Build history of the part. All positions in model axes, mm. Face numbers are marked on the shaded views. A direction names the side the tool comes from. Round coordinates to 2 decimals unless told otherwise and drop trailing zeros. Loops run counter-clockwise (first coordinate to the right, second up) from the corner with the lowest first, then second, coordinate; pieces in that order, holes last. Notation, with made-up numbers: (68, 27.25) - (95, 27.25) arc R23 cw to (95, 49.25) - close; hole circle Ø6 at (-33.75, -31.5). An arc over 180 degrees is marked (long way). Use a Markdown table: item, result.
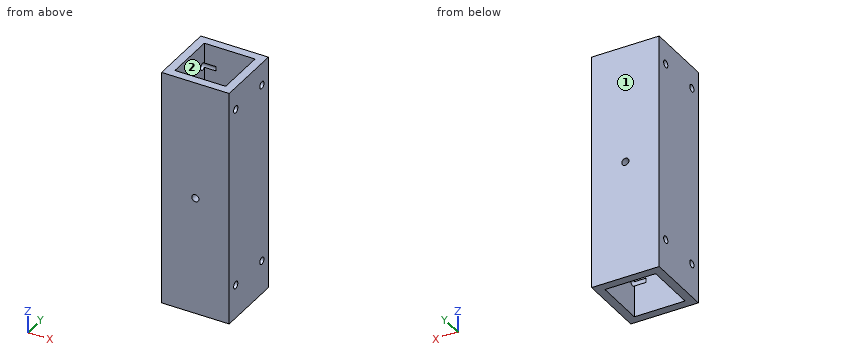
from build123d import *

# Parameters (mm, degrees)
SKETCH1_W                       = 38.1
SKETCH1_H                       = 133.35
BOSS_EXTRUDE1_DEPTH             = 19.05
SKETCH2_W                       = 28.575
SKETCH2_H                       = 28.575
CUT_EXTRUDE1_DEPTH              = 134.35
F_10_32_TAPPED_HOLE1_AT_2_COUNT = 2
F_10_32_TAPPED_HOLE1_AT_2_PITCH = 25.4
F_10_32_TAPPED_HOLE1_AT_3_COUNT = 2
F_10_32_TAPPED_HOLE1_AT_3_PITCH = 104.726882891
F_10_32_TAPPED_HOLE1_AT_4_COUNT = 2
F_10_32_TAPPED_HOLE1_AT_4_PITCH = 101.6
F_10_32_TAPPED_HOLE2_D          = 4.0386


with BuildPart() as part:
    # Sketch1 → Boss-Extrude1 (new body, symmetric)
    with BuildSketch(Plane(origin=(0, 0, 0), x_dir=(1, 0, 0), z_dir=(0, 1, 0))):
        Rectangle(SKETCH1_W, SKETCH1_H)
    extrude(amount=BOSS_EXTRUDE1_DEPTH, both=True)

    # Sketch2 → Cut-Extrude1 (cut, through all)
    with BuildSketch(Plane.XY.offset(66.675)):
        Rectangle(SKETCH2_W, SKETCH2_H)
    extrude(amount=-CUT_EXTRUDE1_DEPTH, mode=Mode.SUBTRACT)

    # Sketch3 → #10-32 Tapped Hole1 (revolve, cut)
    with BuildSketch(Plane(origin=(19.05, -12.7, 53.975), x_dir=(0, 0, -1), z_dir=(0, 1, 0))):
        Polygon((0, 0), (0, 12.389317848), (2.0193, 11.176), (2.0193, 0), align=None)
    f_10_32_tapped_hole1 = revolve(axis=Axis((25.4, -12.7, 53.975), (-1, 0, 0)), mode=Mode.SUBTRACT)

    # #10-32 Tapped Hole1 at 2: #10-32 Tapped Hole1 ×2
    with Locations(*[(0, i * F_10_32_TAPPED_HOLE1_AT_2_PITCH, 0) for i in range(1, F_10_32_TAPPED_HOLE1_AT_2_COUNT)]):
        add(f_10_32_tapped_hole1, mode=Mode.SUBTRACT)

    # #10-32 Tapped Hole1 at 3: #10-32 Tapped Hole1 ×2
    with Locations(*[Vector(0, 0.242535625, -0.9701425) * (i * F_10_32_TAPPED_HOLE1_AT_3_PITCH) for i in range(1, F_10_32_TAPPED_HOLE1_AT_3_COUNT)]):
        add(f_10_32_tapped_hole1, mode=Mode.SUBTRACT)

    # #10-32 Tapped Hole1 at 4: #10-32 Tapped Hole1 ×2
    with Locations(*[(0, 0, -i * F_10_32_TAPPED_HOLE1_AT_4_PITCH) for i in range(1, F_10_32_TAPPED_HOLE1_AT_4_COUNT)]):
        add(f_10_32_tapped_hole1, mode=Mode.SUBTRACT)

    # #10-32 Tapped Hole2 (through all)
    with Locations(Plane(origin=(0, 19.05, 0), x_dir=(1, 0, 0), z_dir=(0, 1, 0))):
        with Locations((0, 0)):
            Hole(F_10_32_TAPPED_HOLE2_D / 2)

    # Mirror1: #10-32 Tapped Hole1 across plane
    add(f_10_32_tapped_hole1.mirror(Plane(origin=(0, 0, 0), x_dir=(0, 0, 1), z_dir=(1, 0, 0))), mode=Mode.SUBTRACT)

    # Mirror1 copy 1 sketch → Mirror1 copy 1 (revolve, cut)
    with BuildSketch(Plane(origin=(-19.05, 12.7, 53.975), x_dir=(0, 0, -1), z_dir=(0, 1, 0))):
        Polygon((0, 0), (0, -12.389317848), (2.0193, -11.176), (2.0193, 0), align=None)
    revolve(axis=Axis((-25.4, 12.7, 53.975), (-1, 0, 0)), mode=Mode.SUBTRACT)

    # Mirror1 copy 2 sketch → Mirror1 copy 2 (revolve, cut)
    with BuildSketch(Plane(origin=(-19.05, 12.7, -47.625), x_dir=(0, 0, -1), z_dir=(0, 1, 0))):
        Polygon((0, 0), (0, -12.389317848), (2.0193, -11.176), (2.0193, 0), align=None)
    revolve(axis=Axis((-25.4, 12.7, -47.625), (-1, 0, 0)), mode=Mode.SUBTRACT)

    # Mirror1 copy 3 sketch → Mirror1 copy 3 (revolve, cut)
    with BuildSketch(Plane(origin=(-19.05, -12.7, -47.625), x_dir=(0, 0, -1), z_dir=(0, 1, 0))):
        Polygon((0, 0), (0, -12.389317848), (2.0193, -11.176), (2.0193, 0), align=None)
    revolve(axis=Axis((-25.4, -12.7, -47.625), (-1, 0, 0)), mode=Mode.SUBTRACT)


solid = part.part
Q1. Which spindle directions (+Z, -Z, +X, -X, +Y, -Y) get a long thin tool onto all of the face, cutting with end or side? Do the marked faces 1 and 2. Say none if no direction does.
Results found:
| item | result |
|---|---|
| face 1 | +Z, -Z, +X, -X, +Y |
| face 2 | +Z, -Z |
Q2. Cut at C-C, the plane z = 0. List the corners of the cut face in (x, y), plus the area to 3 significant figures.
Results found:
| item | result |
|---|---|
| outline | (-19.05, -19.05) - (-2.02, -19.05) - (-2.02, -14.29) - (-14.29, -14.29) - (-14.29, 14.29) - (-2.02, 14.29) - (-2.02, 19.05) - (-19.05, 19.05) - close; (2.02, -19.05) - (19.05, -19.05) - (19.05, 19.05) - (2.02, 19.05) - (2.02, 14.29) - (14.29, 14.29) - (14.29, -14.29) - (2.02, -14.29) - close |
| area | 597 mm2 |
Q3. Cut at A-A, the plane y = 12.7. Count the separate pieces of the cut face and the enclosed holes in it, plus the area to 3 significant figures.
Results found:
| item | result |
|---|---|
| separate pieces | 6 |
| enclosed holes | 0 |
| area | 1,190 mm2 |
Q4. Cut at D-D, the plane z = -21. List the corners of the cut face in (x, y), plus the area to 3 significant figures.
Results found:
| item | result |
|---|---|
| outline | (-19.05, -19.05) - (19.05, -19.05) - (19.05, 19.05) - (-19.05, 19.05) - close; hole (-14.29, -14.29) - (14.29, -14.29) - (14.29, 14.29) - (-14.29, 14.29) - close |
| area | 635 mm2 |
Q5. Probe line 1 (Z direction, x = -15.75, y = 12.7) (3 decimals); line 2 (X direction, y = -8, z = -3). List the from-to ranges inside material, lowest first.
Results found:
| item | result |
|---|---|
| line 1 | z = -66.675 to -49.644, -45.606 to 51.956, 55.994 to 66.675 |
| line 2 | x = -19.05 to -14.29, 14.29 to 19.05 |
